Source: CAD feature listing. Evaluate the final solid. Frame: model axes, mm. A direction names the side the tool comes from. Coordinates: 2 decimals unless noted, no trailing zeros. Order: outer loops, then holes, each group sorted by start corner. A loop starts at its lowest first (then second) coordinate and runs counter-clockwise, first axis right, second up. Notation, with made-up numbers: (-17.5, 78) -> (6.5, 78) arc R33 ccw to (6.5, 114) -> close; hole circle Ø10 at (88.25, 77). An arc over 180 degrees is marked (long way). Write item = value, one per line. Start each with the question number.
Item 1: Section query C-C (z = -34). Output: boundary loops of the cut face in (x, y) (3 decimals).
Item 2: Mould query, pull axis Z, two halves, no side actions, for faces 6 (the flat face through (-1, 19, -82.55)), 7 (the cylindrical face through (-46.367, 3.944, 60.47)), 8 (the flat face through (-47.625, 57, 33)). Classes: released by +Z, released by -Z, zero draft, split by the parting line, or undercut.
Item 3: Section query A-A (x = 0). Count the separate pieces of the cut face and the enclosed holes in it, then the cut area to 3 significant figures.
Item 4: Ray query, line 1 along X through (y, z) = (3.25, 0); line 2 along Z through (x, y) = (17, 72) (3 decimals); line 3 along Y through (x, z) = (-34.5, -60.5). Return the intervals inside material, ascending. Write a range as [from, to].
Item 5: Section query D-D (y = 20.5). Output: boundary loops of the cut face in (x, z).
Item 6: Contact query for flat-ended pins moving along their axis: pin 1 (6 mm diameter, centred on y = 60, z = -33.5, fed in from -X) (3 decimals); pin 2 (23 mm diameter, centred on y = 61.5, z = 29, fed in from +X) (3 decimals); pin 3 (7.5 mm diameter, centred on x = 61.96, z = 61.96, fed in from +Y); pin 4 (1 mm diameter, centred on x = 56, z = 24.5, fed in from +Y). Output: stop coordinate, or through.
Item 7: Set-up query: faces 1 (the flat face through (-1, 91, -19.05)), 2 (the flat face through (-1, 91, -47.625)), 3 (the flat face through (47.625, 57, -33)), 4 (the cylindrical face through (54.2, 27.44, 0.91)), 5 (the cylindrical face through (-25.38, 18.16, 5.64)). Return all of +Z, -Z, +X, -X, +Y, -Y with unobstructed straight access to the full face (end or side cutting, diameter ignored); none if empty.
Item 8: Section query B-B (y = 57). Output: boundary loops of the cut face in (x, z) (3 decimals), then the cut area to 3 significant figures.
```python
from build123d import *

# Parameters (mm, degrees)
SKETCH1_W           = 165.1
SKETCH1_H           = 165.1
SKETCH1_R           = 6.35
BOSS_EXTRUDE1_DEPTH = 38.1
BOSS_EXTRUDE2_START = 19.05
SKETCH2_R           = 12.7
BOSS_EXTRUDE2_DEPTH = 28.575
SKETCH3_R           = 26
CUT_EXTRUDE1_DEPTH  = 36.83
SKETCH4_R           = 7
CUT_EXTRUDE2_DEPTH  = 74.83
CUT_EXTRUDE3_START  = -38.1
CUT_EXTRUDE3_DEPTH  = 17.554240545
FILLET1_R           = 5
SKETCH6_R           = 76.2
SKETCH6_R_2         = 69.85
CUT_EXTRUDE4_DEPTH  = 8


# Read off the part's stored shape, not the designer's step: Cut-Extrude3
with BuildPart() as part:
    # Sketch1 → Boss-Extrude1 (new body)
    with BuildSketch(Plane(origin=(0, 0, 0), x_dir=(1, 0, 0), z_dir=(0, 1, 0))):
        Rectangle(SKETCH1_W, SKETCH1_H)
        with Locations(Location((-61.963767235, 61.963767235, 0), (0, 0, 90))):
            Circle(SKETCH1_R, mode=Mode.SUBTRACT)
        with Locations(Location((61.963767235, 61.963767235, 0), (0, 0, 90))):
            Circle(SKETCH1_R, mode=Mode.SUBTRACT)
        with Locations(Location((61.963767235, -61.963767235, 0), (0, 0, 90))):
            Circle(SKETCH1_R, mode=Mode.SUBTRACT)
        with Locations(Location((-61.963767235, -61.963767235, 0), (0, 0, 90))):
            Circle(SKETCH1_R, mode=Mode.SUBTRACT)
    extrude(amount=BOSS_EXTRUDE1_DEPTH)

    # Sketch2 → Boss-Extrude2 (add)
    with BuildSketch(Plane.XY.offset(BOSS_EXTRUDE2_START)):
        with BuildLine():
            Line((-47.625, 76.2), (-47.625, 38.1))
            Line((-47.625, 38.1), (47.625, 38.1))
            Line((47.625, 38.1), (47.625, 76.2))
            ThreePointArc((47.625, 76.2), (0, 123.825), (-47.625, 76.2))
        make_face()
        with Locations((0, 76.2)):
            Circle(SKETCH2_R, mode=Mode.SUBTRACT)
    boss_extrude2 = extrude(amount=BOSS_EXTRUDE2_DEPTH)

    # Mirror1: Boss-Extrude2 across plane
    add(boss_extrude2.mirror(Plane.XY))

    # Sketch3 → Cut-Extrude1 (cut)
    with BuildSketch(Plane.XZ):
        with Locations(Location((0, 0, 0), (0, 0, 270))):
            Circle(SKETCH3_R)
    extrude(amount=-CUT_EXTRUDE1_DEPTH, mode=Mode.SUBTRACT)

    # Sketch4 → Cut-Extrude2 (cut)
    with BuildSketch(Plane(origin=(82.55, 0, 0), x_dir=(0, 0, -1), z_dir=(1, 0, 0))):
        with Locations((0, 20.5)):
            Circle(SKETCH4_R)
    extrude(amount=-CUT_EXTRUDE2_DEPTH, mode=Mode.SUBTRACT)

    # Cut-Extrude3 outline → Cut-Extrude3 (cut)
    with BuildSketch(Plane(origin=(0, 38.1, 0), x_dir=(1, 0, 0), z_dir=(0, 1, 0)).offset(CUT_EXTRUDE3_START)):
        with BuildLine():
            add(Edge.make_bspline(
                [(50.55, -6.35), (51.47422126, -6.35), (52.302466674, -6.153856691), (53.750900163, -5.540336611), (54.377469866, -5.126654902), (55.505405632, -4.046735856), (55.989700628, -3.386313597), (56.692940175, -1.822566515), (56.897346558, -0.923572623), (56.902599966, 0.886717767), (56.699688489, 1.798962244), (56.004003016, 3.362853664), (55.518127515, 4.030235701), (54.400965604, 5.108341681), (53.760643664, 5.533511906), (52.329554982, 6.145011865), (51.480571337, 6.347463595), (50.110922006, 6.351232148), (49.655780423, 6.301077578), (48.823880157, 6.125660583), (48.443917363, 6.00347472), (47.356446167, 5.544626686), (46.727263651, 5.130170088), (45.598462304, 4.051448232), (45.112857079, 3.390908719), (44.407214336, 1.82399818), (44.202597079, 0.923991808), (44.197454079, -0.88794427), (44.40080252, -1.801200354), (45.098290108, -3.366869707), (45.585297177, -4.034583157), (46.704472395, -5.112538783), (47.346247575, -5.537622225), (48.779720786, -6.147796435), (49.62577874, -6.35), (50.55, -6.35)],
                knots=[0, 0, 0, 0, 0.0625, 0.0625, 0.125, 0.125, 0.1875, 0.1875, 0.25, 0.25, 0.3125, 0.3125, 0.375, 0.375, 0.4375, 0.4375, 0.5, 0.5, 0.53125, 0.53125, 0.5625, 0.5625, 0.625, 0.625, 0.6875, 0.6875, 0.75, 0.75, 0.8125, 0.8125, 0.875, 0.875, 0.9375, 0.9375, 1, 1, 1, 1], degree=3))
        make_face()
    extrude(amount=CUT_EXTRUDE3_DEPTH, mode=Mode.SUBTRACT)

    # Fillet1
    fillet1_edges = [part.edges().sort_by_distance(p)[0] for p in [
        (82.55, 19.05, 82.55),
        (-82.55, 19.05, 82.55),
        (-82.55, 19.05, -82.55),
        (82.55, 19.05, -82.55),
    ]]
    fillet(fillet1_edges, radius=FILLET1_R)

    # Sketch6 → Cut-Extrude4 (cut)
    with BuildSketch(Plane.XZ):
        with Locations(Location((0, 0, 0), (0, 0, 270))):
            Circle(SKETCH6_R)
        with Locations(Location((0, 0, 0), (0, 0, 270))):
            Circle(SKETCH6_R_2, mode=Mode.SUBTRACT)
    extrude(amount=-CUT_EXTRUDE4_DEPTH, mode=Mode.SUBTRACT)


solid = part.part
```
Computed:
q1.outline = (-82.55, 0) -> (-68.194, 0) -> (-68.194, 8) -> (-61.017, 8) -> (-61.017, 0) -> (61.017, 0) -> (61.017, 8) -> (68.194, 8) -> (68.194, 0) -> (82.55, 0) -> (82.55, 38.1) -> (47.625, 38.1) -> (47.625, 76.2) arc R47.625 ccw to (-47.625, 76.2) -> (-47.625, 38.1) -> (-82.55, 38.1) -> close; hole circle Ø25.4 at (0, 76.2)
q2.face_6 = released by -Z
q2.face_7 = undercut
q2.face_8 = zero draft
q3.separate_pieces = 3
q3.enclosed_holes = 0
q3.area = 7,720 mm^2
q4.line_1 = [-82.55, -76.2], [-69.85, -26], [26, 44.2], [56.9, 69.85], [76.2, 82.55]
q4.line_2 = [-47.625, -19.05], [19.05, 47.625]
q4.line_3 = [0, 38.1]
q5.outline = (-82.55, -77.55) arc R5 ccw to (-77.55, -82.55) -> (77.55, -82.55) arc R5 ccw to (82.55, -77.55) -> (82.55, -7) -> (25.04, -7) arc R26 cw (long way) to (25.04, 7) -> (82.55, 7) -> (82.55, 77.55) arc R5 ccw to (77.55, 82.55) -> (-77.55, 82.55) arc R5 ccw to (-82.55, 77.55) -> close; hole circle Ø12.7 at (-61.96, -61.96); hole circle Ø12.7 at (-61.96, 61.96); hole circle Ø12.7 at (61.96, -61.96); hole circle Ø12.7 at (61.96, 61.96)
q6.pin_1 = -47.625
q6.pin_2 = 47.625
q6.pin_3 = through
q6.pin_4 = 38.1
q7.face_1 = +X, -X, +Y
q7.face_2 = -Z, +X, -X, +Y
q7.face_3 = +Z, -Z, +X, +Y
q7.face_4 = +X
q7.face_5 = -Y
q8.outline = (-47.625, -47.625) -> (47.625, -47.625) -> (47.625, -19.05) -> (-47.625, -19.05) -> close; (-47.625, 19.05) -> (47.625, 19.05) -> (47.625, 47.625) -> (-47.625, 47.625) -> close
q8.area = 5,440 mm^2
